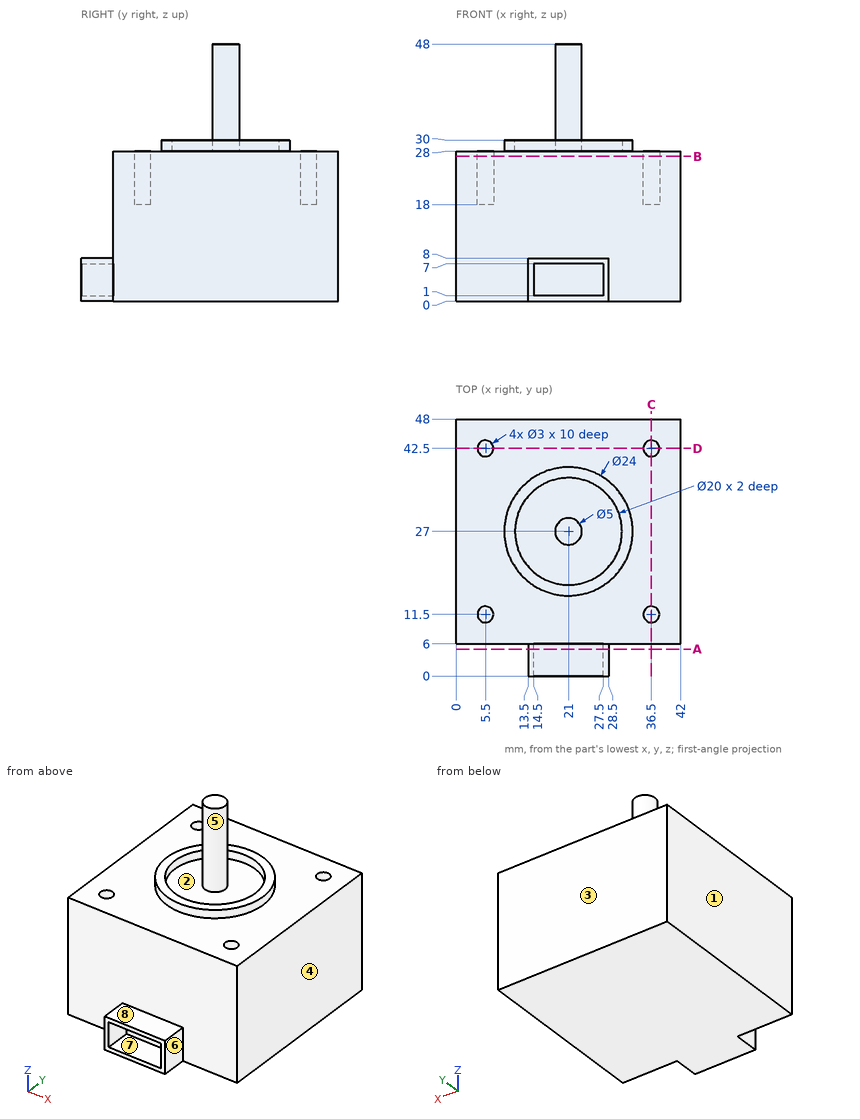
Can you work these out from the drawing? Everything is in mm from the part's minimum corner. A direction names the side the tool comes from. Coordinates: 2 decimals unless noted, no trailing zeros. Loops run counter-clockwise (first coordinate to the right, second up) from the corner with the lowest first, then second, coordinate; pieces in that order, holes last.
1) I need wall thicknesses on probe 1 along Y at (x, z) = (5.5, 22.25); probe 2 along Y at (x, z) = (21, 28.4); probe 3 along X at (y, z) = (42, 25). Which ranges of each line are inside material? Lowest first, please.
2) Imagine slicing it at A-A on y = 5. List the corners of the cut face in (x, z) for me.
3) For pin 1 (1.5 mm diameter, centred on x = 5, y = 11.5, fed in from +Z); pin 2 (3.5 mm diameter, centred on x = 36.5, y = 42.5, fed in from +Z); pin 3 (8.5 mm diameter, centred on x = 13, z = 19, fed in from -Y), each with a flat end and sliding along its axis, tell me the tip position at first contact or that it passes through.
4) Imagine slicing it at C-C on x = 36.5. List the corners of the cut face in (y, z) for me, plus the area to 3 significant figures.
5) Imagine slicing it at D-D on y = 42.5. List the corners of the cut face in (x, z) for me.
6) Thinking about a two-plate mould opening in X: for the marked faces 1, 2 and 3, which applies, pulls with the +X half, pulls with the -X half, needs draft (parallel to the pull), parting line crosses it, or undercut?
7) Which directions (+Z, -Z, +X, -X, +Y, -Y) give clear straight access to the entire face, cutting with the end or side of a thin tool? Please do the marked faces 4, 5, 6, 7 and 8.
8) Imagine slicing it at B-B on z = 27. List the corners of the cut face in (x, y) for me, plus the area to 3 significant figures.
Completed:
1. probe 1: y = 6 to 10, 13 to 41, 44 to 48
1. probe 2: y = 15 to 17, 24.5 to 29.5, 37 to 39
1. probe 3: x = 0 to 4.09, 6.91 to 35.09, 37.91 to 42
2. outline: (13.5, 0) - (28.5, 0) - (28.5, 8) - (13.5, 8) - close; hole (14.5, 1) - (27.5, 1) - (27.5, 7) - (14.5, 7) - close
3. pin 1: stops at z = 18
3. pin 2: stops at z = 28
3. pin 3: stops at y = 6
4. outline: (6, 0) - (48, 0) - (48, 28) - (44, 28) - (44, 18) - (41, 18) - (41, 28) - (13, 28) - (13, 18) - (10, 18) - (10, 28) - (6, 28) - close
4. area: 1,120 mm2
5. outline: (0, 0) - (42, 0) - (42, 28) - (38, 28) - (38, 18) - (35, 18) - (35, 28) - (7, 28) - (7, 18) - (4, 18) - (4, 28) - (0, 28) - close
6. face 1: pulls with the -X half
6. face 2: undercut
6. face 3: needs draft
7. face 4: +Z, -Z, +X, +Y, -Y
7. face 5: +Z
7. face 6: +Z, -Z, +X, -Y
7. face 7: -Y
7. face 8: +Z, +X, -X, -Y
8. outline: (0, 6) - (42, 6) - (42, 48) - (0, 48) - close; hole circle Ø3 at (5.5, 11.5); hole circle Ø3 at (5.5, 42.5); hole circle Ø3 at (36.5, 11.5); hole circle Ø3 at (36.5, 42.5)
8. area: 1,740 mm2
